```python
from build123d import *

# Parameters (mm, degrees)
SKETCH2_R             = 2
BOSS_EXTRUDE2_DEPTH   = 5
BOSS_EXTRUDE2_2_DEPTH = 5
BOSS_EXTRUDE2_3_DEPTH = 5
SKETCH3_W             = 194
SKETCH3_H             = 156
BOSS_EXTRUDE3_DEPTH   = 10
SKETCH5_R             = 2
BOSS_EXTRUDE4_DEPTH   = 10
SKETCH6_W             = 80.829037686
SKETCH6_H             = 10
CUT_EXTRUDE1_DEPTH    = 142
SKETCH7_R             = 2
CUT_EXTRUDE2_DEPTH    = 142
CUT_EXTRUDE4_DEPTH    = 10
BOSS_EXTRUDE5_DEPTH   = 20
SKETCH10_R            = 2
CUT_EXTRUDE5_DEPTH    = 1
CUT_EXTRUDE6_DEPTH    = 1
BOSS_EXTRUDE6_DEPTH   = 5
BOSS_EXTRUDE7_DEPTH   = 5


with BuildPart() as part:
    # Sketch2 → Boss-Extrude2 (new, symmetric)
    with BuildSketch(Plane.XY):
        with BuildLine():
            ThreePointArc((50.330127019, 12.5), (46, 15), (41.669872981, 12.5))
            Line((41.669872981, 12.5), (5.585481157, -50))
            Line((5.585481157, -50), (86.414518843, -50))
            Line((86.414518843, -50), (50.330127019, 12.5))
        make_face()
        with Locations((46, 10)):
            Circle(SKETCH2_R, mode=Mode.SUBTRACT)
    extrude(amount=BOSS_EXTRUDE2_DEPTH, both=True)



with BuildPart() as body_2:
    # Sketch2 → Boss-Extrude2 2 (new, symmetric)
    with BuildSketch(Plane.XY):
        with BuildLine():
            Line((-21.547005384, -50), (1.547005384, -50))
            Line((1.547005384, -50), (-5.669872981, -37.5))
            ThreePointArc((-5.669872981, -37.5), (-10, -35), (-14.330127019, -37.5))
            Line((-14.330127019, -37.5), (-21.547005384, -50))
        make_face()
        with Locations((-10, -40)):
            Circle(SKETCH2_R, mode=Mode.SUBTRACT)
    extrude(amount=BOSS_EXTRUDE2_2_DEPTH, both=True)


with BuildPart() as body_3:
    # Sketch2 → Boss-Extrude2 3 (new, symmetric)
    with BuildSketch(Plane.XY):
        with BuildLine():
            Line((-88.331615075, -50), (-23.668384925, -50))
            Line((-23.668384925, -50), (-51.669872981, -1.5))
            ThreePointArc((-51.669872981, -1.5), (-56, 1), (-60.330127019, -1.5))
            Line((-60.330127019, -1.5), (-88.331615075, -50))
        make_face()
        with Locations((-56, -4)):
            Circle(SKETCH2_R, mode=Mode.SUBTRACT)
    extrude(amount=BOSS_EXTRUDE2_3_DEPTH, both=True)


with BuildPart() as part_1:
    add(part.part)

    add(body_2.part)  # Boss-Extrude3 merges body 2

    add(body_3.part)  # Boss-Extrude3 merges body 3
    # Sketch3 → Boss-Extrude3 (add)
    with BuildSketch(Plane(origin=(0, -50, 0), x_dir=(-1, 0, 0), z_dir=(0, -1, 0))):
        Rectangle(SKETCH3_W, SKETCH3_H)
    extrude(amount=BOSS_EXTRUDE3_DEPTH)

    # Sketch5 → Boss-Extrude4 (add)
    # profile 1 of 3: a face of its own
    with BuildSketch(Plane.XY.offset(15)):
        with BuildLine():
            Line((-88.331615075, -50), (-23.668384925, -50))
            Line((-23.668384925, -50), (-51.669872981, -1.5))
            ThreePointArc((-51.669872981, -1.5), (-56, 1), (-60.330127019, -1.5))
            Line((-60.330127019, -1.5), (-88.331615075, -50))
        make_face()
        with Locations((-56, -4)):
            Circle(SKETCH5_R, mode=Mode.SUBTRACT)
    # profile 2 of 3: a face of its own
    with BuildSketch(Plane.XY.offset(15)):
        with BuildLine():
            Line((-21.547005384, -50), (1.547005384, -50))
            Line((1.547005384, -50), (-5.669872981, -37.5))
            ThreePointArc((-5.669872981, -37.5), (-10, -35), (-14.330127019, -37.5))
            Line((-14.330127019, -37.5), (-21.547005384, -50))
        make_face()
        with Locations((-10, -40)):
            Circle(SKETCH5_R, mode=Mode.SUBTRACT)
    # profile 3 of 3: a face of its own
    with BuildSketch(Plane.XY.offset(15)):
        with BuildLine():
            ThreePointArc((50.330127019, 12.5), (46, 15), (41.669872981, 12.5))
            Line((41.669872981, 12.5), (5.585481157, -50))
            Line((5.585481157, -50), (86.414518843, -50))
            Line((86.414518843, -50), (50.330127019, 12.5))
        make_face()
        with Locations((46, 10)):
            Circle(SKETCH5_R, mode=Mode.SUBTRACT)
    boss_extrude4 = extrude(amount=BOSS_EXTRUDE4_DEPTH)

    # Mirror1: Boss-Extrude4 across plane
    add(boss_extrude4.mirror(Plane.XY))

    # Sketch6 → Cut-Extrude1 (cut)
    with BuildSketch(Plane(origin=(0, -50, 0), x_dir=(1, 0, 0), z_dir=(0, 1, 0))):
        with Locations((46, 0)):
            Rectangle(SKETCH6_W, SKETCH6_H)
    extrude(amount=CUT_EXTRUDE1_DEPTH, mode=Mode.SUBTRACT)

    # Sketch7 → Cut-Extrude2 (cut)
    with BuildSketch(Plane(origin=(0, -50, 0), x_dir=(1, 0, 0), z_dir=(0, 1, 0))):
        with Locations(Location((-92, -73, 0), (0, 0, 270))):
            Circle(SKETCH7_R)
        with Locations(Location((-92, 73, 0), (0, 0, 270))):
            Circle(SKETCH7_R)
        with Locations(Location((92, 73, 0), (0, 0, 270))):
            Circle(SKETCH7_R)
        with Locations(Location((92, -73, 0), (0, 0, 270))):
            Circle(SKETCH7_R)
    extrude(amount=-CUT_EXTRUDE2_DEPTH, mode=Mode.SUBTRACT)

    # Sketch8 → Cut-Extrude4 (cut)
    with BuildSketch(Plane.XY.offset(25)):
        Polygon((-71, -7), (-41, -7), (-41, -1), (-41, 3.028567104), (-71, 3.028567104), (-71, -1), align=None)
    extrude(amount=-CUT_EXTRUDE4_DEPTH, mode=Mode.SUBTRACT)

    # Sketch9 → Boss-Extrude5 (add)
    with BuildSketch(Plane.XY.offset(25)):
        Polygon((-88.331615075, -50), (-23.668384925, -50), (-48.494446501, -7), (-63.505553499, -7), align=None)
    extrude(amount=BOSS_EXTRUDE5_DEPTH)

    # Sketch10 → Cut-Extrude5 (cut)
    # profile 1 of 2: a face of its own
    with BuildSketch(Plane.XY.offset(5)):
        with BuildLine():
            Line((-60.330127019, -1.5), (-88.331615075, -50))
            Line((-88.331615075, -50), (-23.668384925, -50))
            Line((-23.668384925, -50), (-51.669872981, -1.5))
            ThreePointArc((-51.669872981, -1.5), (-56, 1), (-60.330127019, -1.5))
        make_face()
        with Locations((-56, -4)):
            Circle(SKETCH10_R, mode=Mode.SUBTRACT)
    # profile 2 of 2: a face of its own
    with BuildSketch(Plane.XY.offset(5)):
        with BuildLine():
            Line((-21.547005384, -50), (-14.330127019, -37.5))
            ThreePointArc((-14.330127019, -37.5), (-10, -35), (-5.669872981, -37.5))
            Line((-5.669872981, -37.5), (1.547005384, -50))
            Line((1.547005384, -50), (-21.547005384, -50))
        make_face()
    cut_extrude5 = extrude(amount=-CUT_EXTRUDE5_DEPTH, mode=Mode.SUBTRACT)

    # Mirror2: Cut-Extrude5 across plane
    add(cut_extrude5.mirror(Plane.XY), mode=Mode.SUBTRACT)

    # Sketch11 → Cut-Extrude6 (cut)
    with BuildSketch(Plane.XY.offset(-15)):
        with BuildLine():
            Line((-88.331615075, -50), (-23.668384925, -50))
            Line((-23.668384925, -50), (-51.669872981, -1.5))
            ThreePointArc((-51.669872981, -1.5), (-56, 1), (-60.330127019, -1.5))
            Line((-60.330127019, -1.5), (-88.331615075, -50))
        make_face()
        with BuildLine():
            Line((-21.547005384, -50), (1.547005384, -50))
            Line((1.547005384, -50), (-5.669872981, -37.5))
            ThreePointArc((-5.669872981, -37.5), (-10, -35), (-14.330127019, -37.5))
            Line((-14.330127019, -37.5), (-21.547005384, -50))
        make_face()
        with BuildLine():
            Line((5.585481157, -50), (41.669872981, 12.5))
            ThreePointArc((41.669872981, 12.5), (46, 15), (50.330127019, 12.5))
            Line((50.330127019, 12.5), (86.414518843, -50))
            Line((86.414518843, -50), (5.585481157, -50))
        make_face()
    cut_extrude6 = extrude(amount=-CUT_EXTRUDE6_DEPTH, mode=Mode.SUBTRACT)

    # Mirror3: Cut-Extrude6 across plane
    add(cut_extrude6.mirror(Plane.XY), mode=Mode.SUBTRACT)

    # Sketch12 → Boss-Extrude6 (add, symmetric)
    with BuildSketch(Plane(origin=(46, 0, 0), x_dir=(0, 0, -1), z_dir=(1, 0, 0))):
        Polygon((-55, -50), (-25, -10), (-25, -50), align=None)
    boss_extrude6 = extrude(amount=BOSS_EXTRUDE6_DEPTH, both=True)

    # Mirror4: Boss-Extrude6 across plane
    add(boss_extrude6.mirror(Plane.XY))

    # Sketch13 → Boss-Extrude7 (add, symmetric)
    with BuildSketch(Plane.ZY.offset(56)):
        Polygon((-45, -50), (-25, -23.333333333), (-25, -50), align=None)
    extrude(amount=BOSS_EXTRUDE7_DEPTH, both=True)


solid = part_1.part
```
The listing builds one solid part. Answer for the finished solid, in the listing's coordinates (mm). A direction names the side the tool comes from. Round coordinates to 2 decimals unless told otherwise and drop trailing zeros. Loops run counter-clockwise (first coordinate to the right, second up) from the corner with the lowest first, then second, coordinate; pieces in that order, holes last.
1) A cutting plane is placed at C-C on z = 41. Determine the outline of the cut face in (x, y), plus the area to 3 significant figures.
Outcome:
outline: (-97, -60) - (97, -60) - (97, -50) - (51, -50) - (51, -31.33) - (41, -31.33) - (41, -50) - (-23.67, -50) - (-48.49, -7) - (-63.51, -7) - (-88.33, -50) - (-97, -50) - close
area: 3,840 mm2
2) A cutting plane is placed at B-B on x = 8. Determine the outline of the cut face in (y, z).
Outcome:
outline: (-60, -78) - (-50, -78) - (-50, -25) - (-45.82, -25) - (-45.82, -16) - (-50, -16) - (-50, 16) - (-45.82, 16) - (-45.82, 25) - (-50, 25) - (-50, 78) - (-60, 78) - close
3) For faces 5 (the face through (51, -39, -33)), 6 (the face through (-61, -42, -30)), 7 (the face through (-51, -42, -30)), determine the directions among +Z, -Z, +X, -X, +Y, -Y from which every point of the face is accessible in a straight line to the end or side of a thin tool.
Outcome:
face 5: -Z, +X, +Y
face 6: -Z, -X, +Y
face 7: -Z, +Y
4) A cutting plane is placed at A-A on y = -31.5. Give the number of separate pieces and of enclosed holes in the cut face, plus the area to 3 significant figures.
Outcome:
separate pieces: 5
enclosed holes: 0
area: 3,450 mm2
5) Consider line 1 (X direction, y = -55, z = 73); line 2 (Y direction, x = 46, z = 21); line 3 (Z direction, x = 54, y = -2). Determine where each line is inside the solid, lowest interval first.
Outcome:
line 1: x = -97 to -94, -90 to 90, 94 to 97
line 2: y = -60 to 8, 12 to 15
line 3: z = -25 to -16, 16 to 25
6) Given P1, Ø6, axis at x = 71.5, y = -44.5, coming from the -Z side; P2, Ø15, axis at y = -25, z = -43.5, coming from the -X side; P3, Ø2.5, axis at x = -10, y = -40, coming from the -Z side; P4, Ø9, axis at y = -33, z = -38.5, coming from the +X side, each flat-ended and moving along its own axis, determine where each tip first touches the part or whether it passes through.
Outcome:
P1: stops at z = -25
P2: stops at x = 41
P3: passes through
P4: stops at x = 51
7) A cutting plane is placed at D-D on x = -69. Determine the outline of the cut face in (y, z).
Outcome:
outline: (-60, -78) - (-50, -78) - (-50, -25) - (-16.52, -25) - (-16.52, -16) - (-50, -16) - (-50, -4) - (-16.52, -4) - (-16.52, 4) - (-50, 4) - (-50, 16) - (-16.52, 16) - (-16.52, 45) - (-50, 45) - (-50, 78) - (-60, 78) - close
8) For a pull along Z with two mould halves and no side action, classify faces 1 (the face through (-10, -44, 25)), 2 (the face through (47, -24, 16)), 3 (the face through (-49, -30, -25)), 4 (the face through (-2.01, -43.84, -20.44)) as released by +Z, released by -Z, zero draft, split by the parting line, or undercut.
Outcome:
face 1: released by +Z
face 2: undercut
face 3: released by -Z
face 4: zero draft
